Geometry check sheet. Reference: the model listing, model coordinates, mm. Round coordinates to 2 decimals unless told otherwise and drop trailing zeros. Order: outer loops, then holes, each group sorted by start corner. A loop starts at its lowest first (then second) coordinate and runs counter-clockwise, first axis right, second up. Notation, with made-up numbers: (33.5, -37) - (52.5, -37) arc R11 ccw to (52.5, -25) - close; hole circle Ø6 at (45.25, -6.75). An arc over 180 degrees is marked (long way). Use a Markdown table: item, result. Add a question column.
(1) Section check D-D on x = 93.5. Record the boundary of the cut face in (y, z) (3 decimals).
(2) Section check C-C on z = 138.5. Record the boundary of the cut face in (x, y) (3 decimals).
(3) Gauge pin test, flat end, axial feed: P1, Ø3, axis at x = 35, y = 4.5, coming from the +Z side. Record the tip position at first contact, or that the pin passes through.
(4) Thickness scan on line 1 along Z through (x, y) = (134, 16.25); line 2 along Z through (x, y) = (100.5, 13); line 3 along X through (y, z) = (10.75, 129) (3 decimals). Record the ranges inside material, lowest first. Write a range as [from, to].
(5) Section check A-A on y = 14.75. Record the boundary of the cut face in (x, z) (3 decimals), then the cut area to 3 significant figures.
(6) Section check B-B on x = 170. Record the boundary of the cut face in (y, z) (3 decimals).
```python
from build123d import *

# Parameters (mm, degrees)
SKETCH1_W           = 346.7
SKETCH1_H           = 357.50000001
BOSS_EXTRUDE1_DEPTH = 18
SKETCH2_W           = 346.7
SKETCH2_H           = 18
CUT_EXTRUDE1_DEPTH  = 6.35
SKETCH3_W           = 133.35
SKETCH3_H           = 107.95
CUT_EXTRUDE3_DEPTH  = 19
FILLET1_R           = 9.525


with BuildPart() as part:
    # Sketch1 → Boss-Extrude1 (new body)
    with BuildSketch(Plane(origin=(0, 0, 0), x_dir=(1, 0, 0), z_dir=(0, 1, 0))):
        with Locations((173.35, -178.750000005)):
            Rectangle(SKETCH1_W, SKETCH1_H)
    extrude(amount=BOSS_EXTRUDE1_DEPTH)

    # Sketch2 → Cut-Extrude1 (cut)
    with BuildSketch(Plane(origin=(0, 18, 0), x_dir=(1, 0, 0), z_dir=(0, 1, 0))):
        with Locations((173.35, -310.40000001)):
            Rectangle(SKETCH2_W, SKETCH2_H)
    extrude(amount=-CUT_EXTRUDE1_DEPTH, mode=Mode.SUBTRACT)

    # Sketch3 → Cut-Extrude3 (cut, through all)
    with BuildSketch(Plane(origin=(0, 18, 0), x_dir=(1, 0, 0), z_dir=(0, 1, 0))):
        with Locations((173.35, -176.52500001)):
            Rectangle(SKETCH3_W, SKETCH3_H)
    extrude(amount=-CUT_EXTRUDE3_DEPTH, mode=Mode.SUBTRACT)

    # Fillet1
    fillet1_edges = [part.edges().sort_by_distance(p)[0] for p in [
        (173.35, 0, 357.50000001),
    ]]
    fillet(fillet1_edges, radius=FILLET1_R)


solid = part.part
```
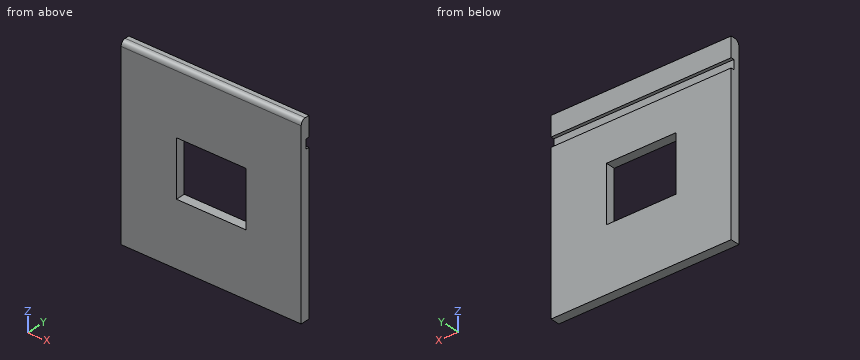
Check sheet entries:
| question | item | result |
|---|---|---|
| 1 | outline | (0, 0) - (18, 0) - (18, 301.4) - (11.65, 301.4) - (11.65, 319.4) - (18, 319.4) - (18, 357.5) - (9.525, 357.5) arc R9.525 ccw to (0, 347.975) - close |
| 2 | outline | (0, 0) - (106.675, 0) - (106.675, 18) - (0, 18) - close; (240.025, 0) - (346.7, 0) - (346.7, 18) - (240.025, 18) - close |
| 3 | P1 | stops at z = 356.82 |
| 4 | line 1 | z = [0, 122.55], [230.5, 301.4], [319.4, 357.5] |
| 4 | line 2 | z = [0, 301.4], [319.4, 357.5] |
| 4 | line 3 | x = [0, 106.675], [240.025, 346.7] |
| 5 | outline | (0, 0) - (346.7, 0) - (346.7, 301.4) - (0, 301.4) - close; (0, 319.4) - (346.7, 319.4) - (346.7, 357.5) - (0, 357.5) - close; hole (106.675, 122.55) - (240.025, 122.55) - (240.025, 230.5) - (106.675, 230.5) - close |
| 5 | area | 103,000 mm2 |
| 6 | outline | (0, 0) - (18, 0) - (18, 122.55) - (0, 122.55) - close; (0, 230.5) - (18, 230.5) - (18, 301.4) - (11.65, 301.4) - (11.65, 319.4) - (18, 319.4) - (18, 357.5) - (9.525, 357.5) arc R9.525 ccw to (0, 347.975) - close |
